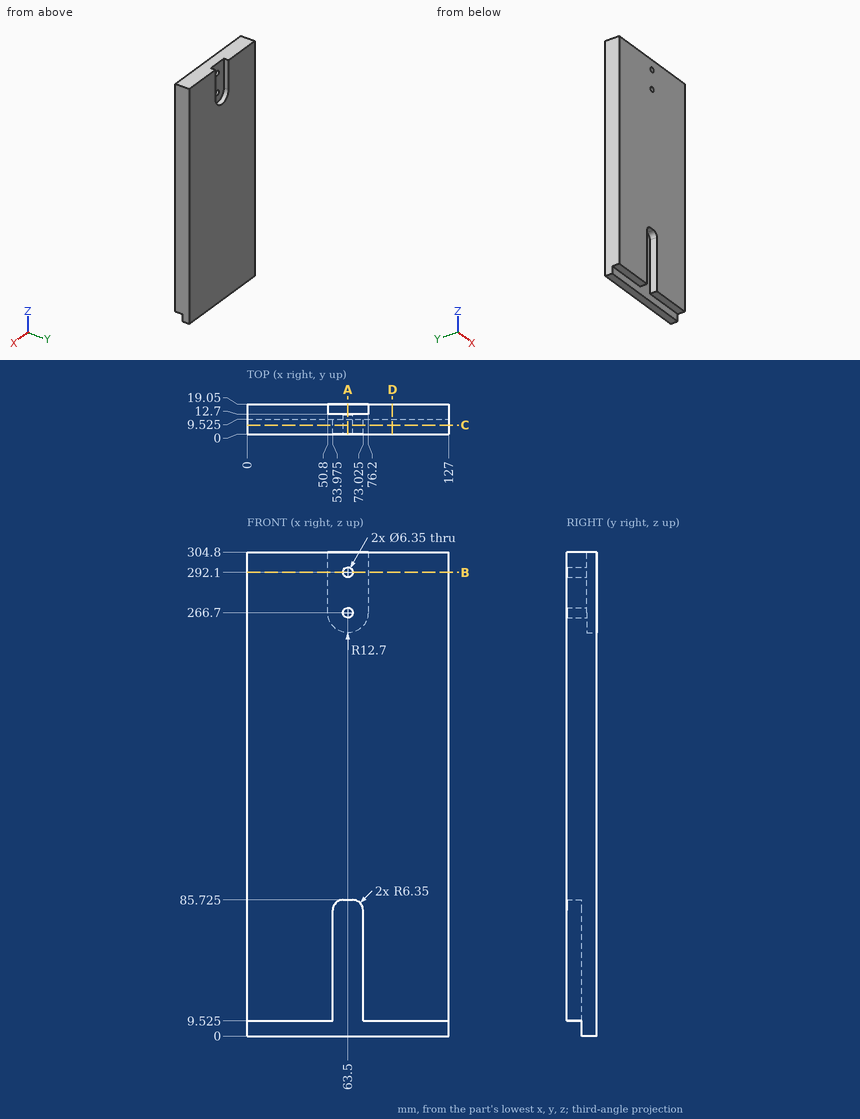
Here's the drawing with two shaded views (mm, measured from the low corner). I have some questions. Coordinates: 2 decimals unless noted, no trailing zeros. Write each loop counter-clockwise with the first axis right and the second up, starting at its lowest first coordinate (ties: lowest second). Pieces come first, ordered by that corner, then holes.
Item 1: I want a section at A-A on x = 63.5. Write out the boundary of the cut face in (y, z) (3 decimals).
Item 2: If I drill on line 1 (Z direction, x = 63.5, y = 6.25) (3 decimals); line 2 (X direction, y = 7, z = 266.7) (3 decimals); line 3 (X direction, y = 5.5, z = 18.5) (3 decimals), over which ranges is the centre line in solid material (lowest first)?
Item 3: I want a section at D-D on x = 91.5. Write out the boundary of the cut face in (y, z) (3 decimals).
Item 4: I want a section at C-C on y = 5.75. Write out the boundary of the cut face in (x, z) (3 decimals).
Item 5: I want a section at B-B on z = 292.1. Write out the boundary of the cut face in (x, y) (3 decimals), and give its area (3 significant figures).
Item 6: Will these pins go through, and if not, where does the flat tip stop? pin 1 (3 mm diameter, centred on x = 68, z = 259.5, fed in from +Y); pin 2 (3 mm diameter, centred on x = 109.5, y = 6, fed in from -Z) (3 decimals); pin 3 (3 mm diameter, centred on x = 64.5, y = 5.5, fed in from -Z) (3 decimals).
Findings below:
1. outline: (0, 85.725) - (9.525, 85.725) - (9.525, 0) - (19.05, 0) - (19.05, 254) - (12.7, 254) - (12.7, 263.525) - (0, 263.525) - close; (0, 269.875) - (12.7, 269.875) - (12.7, 288.925) - (0, 288.925) - close; (0, 295.275) - (12.7, 295.275) - (12.7, 304.8) - (0, 304.8) - close
2. line 1: z = 85.725 to 263.525, 269.875 to 288.925, 295.275 to 304.8
2. line 2: x = 0 to 60.325, 66.675 to 127
2. line 3: x = 0 to 53.975, 73.025 to 127
3. outline: (0, 9.525) - (9.525, 9.525) - (9.525, 0) - (19.05, 0) - (19.05, 304.8) - (0, 304.8) - close
4. outline: (0, 9.525) - (53.975, 9.525) - (53.975, 79.375) arc R6.35 cw to (60.325, 85.725) - (66.675, 85.725) arc R6.35 cw to (73.025, 79.375) - (73.025, 9.525) - (127, 9.525) - (127, 304.8) - (0, 304.8) - close; hole circle Ø6.35 at (63.5, 266.7); hole circle Ø6.35 at (63.5, 292.1)
5. outline: (0, 0) - (60.325, 0) - (60.325, 12.7) - (50.8, 12.7) - (50.8, 19.05) - (0, 19.05) - close; (66.675, 0) - (127, 0) - (127, 19.05) - (76.2, 19.05) - (76.2, 12.7) - (66.675, 12.7) - close
5. area: 2,180 mm2
6. pin 1: stops at y = 12.7
6. pin 2: stops at z = 9.525
6. pin 3: stops at z = 85.725
